from build123d import *

# Parameters (mm, degrees)
F2_SIZE        = 0.5
F4_DEPTH       = 2.5
F6_D           = 6.5
F6_CBORE_D     = 10.5
F6_CBORE_DEPTH = 5


with BuildPart() as f1:
    # F0 (on Top) → F1 (revolve)
    with BuildSketch(Plane.XY):
        with BuildLine():
            Line((-47.750211, -7.25), (-47.750212, -8))
            Line((-47.750212, -8), (-25.000581, -8))
            Line((-25.000581, -8), (-25, 0))
            Line((-25, 0), (-47.75, 0))
            Line((-47.75, 0), (-47.75019, -4))
            Line((-47.75019, -4), (-47.250211, -4))
            ThreePointArc((-47.250211, -4), (-46.189551, -4.43934), (-45.750211, -5.5))
            Line((-45.750211, -5.5), (-45.750211, -5.75))
            ThreePointArc((-45.750211, -5.75), (-46.189551, -6.81066), (-47.250211, -7.25))
            Line((-47.250211, -7.25), (-47.750211, -7.25))
        make_face()
    revolve(axis=Axis((0, 4.349666, 0), (0, 1, 0)))

    # F2
    f2_edges = [f1.edges().sort_by_distance(p)[0] for p in [
        (25.000581, -8, 0),
    ]]
    chamfer(f2_edges, length=F2_SIZE)

    # F3 (on face) → F4 (cut)
    with BuildSketch(Plane(origin=(0, 0, 0), x_dir=(-1, 0, 0), z_dir=(0, 1, 0))):
        with BuildLine():
            ThreePointArc((-4.265587, -23.938974), (-7.351028, -20.725712), (-10.56429, -23.811154))
            Line((-10.56429, -23.811154), (-11.035483, -47.030372))
            ThreePointArc((-11.035483, -47.030372), (-7.950042, -50.243634), (-4.73678, -47.158193))
            Line((-4.73678, -47.158193), (-4.265587, -23.938974))
        make_face()
    extrude(amount=-F4_DEPTH, mode=Mode.SUBTRACT)

    # F6 (through all)
    with Locations(Plane.XZ.offset(8)):
        with Locations((-28.85, 13.73333), (27.356101, 15.955209), (-0.6, -31.7)):
            CounterBoreHole(F6_D / 2, F6_CBORE_D / 2, F6_CBORE_DEPTH)


solid = f1.part
The listing builds one solid part. Answer for the finished solid, in the listing's coordinates (mm). A direction names the side the tool comes from. Coordinates: 2 decimals unless noted, no trailing zeros. Write each loop counter-clockwise with the first axis right and the second up, starting at its lowest first coordinate (ties: lowest second). Pieces come first, ordered by that corner, then holes. Notation, with made-up numbers: (49.25, 28) -> (87.25, 28) arc R8 cw to (87.25, 36) -> close; hole circle Ø9 at (83.25, 14.25). An arc over 180 degrees is marked (long way). One line per question, with ' | ' between items.
1. Which of the six approach directions +Z, -Z, +X, -X, +Y, -Y give full straight-line access (tool end or side, diameter ignored) to faces 1 (the flat face through (-21, -8, -21)), 2 (the cylindrical face through (32.206, -5.535, 13.944)), 3 (the flat face through (-46.2, -7.25, 10.8))?
Verdict:
face 1: +Z, -Z, +X, -X, -Y | face 2: -Y | face 3: none
2. For a pull along Y with two mould halves and no side action, classify faces 4 (the cylindrical face through (-23.842, -5.535, 15.31)), 5 (the flat face through (10.8, -4, 46.2)), 6 (the flat face through (21, 0, 22)) as released by +Y, released by -Y, zero draft, split by the parting line, or undercut.
Verdict:
face 4: zero draft | face 5: undercut | face 6: released by +Y
3. Section A-A (z = 0) is taken. Determine the outline of the cut face in (x, y).
Verdict:
outline: (-47.75, -8) -> (-25.5, -8) -> (-25, -7.5) -> (-25, 0) -> (-47.75, 0) -> (-47.75, -4) -> (-47.25, -4) arc R1.5 cw to (-45.75, -5.5) -> (-45.75, -5.75) arc R1.5 cw to (-47.25, -7.25) -> (-47.75, -7.25) -> close; (25, -7.5) -> (25.5, -8) -> (47.75, -8) -> (47.75, -7.25) -> (47.25, -7.25) arc R1.5 cw to (45.75, -5.75) -> (45.75, -5.5) arc R1.5 cw to (47.25, -4) -> (47.75, -4) -> (47.75, 0) -> (25, 0) -> close
4. Given pin 1 Ø1.5 at (y, z) = (-1.5, -15) entering from -X; pin 2 Ø3 at (x, y) = (24, -7) entering from +Z; pin 3 Ø3 at (x, z) = (0.5, -29.5) entering from -Y, each flat-ended and moving along its own axis, determine where each tip first touches the part or whether it passes through.
Verdict:
pin 1: stops at x = -45.57 | pin 2: stops at z = 42.11 | pin 3: stops at y = -3
5. Straight lines are drawn through the part: line 1 (Z direction, x = -0.6, y = -1.2); line 2 (Z direction, x = -0.6, y = -5.1); line 3 (Z direction, x = -15, y = -2.25). For each, find the intervals that lie inside material, in ascending order.
Verdict:
line 1: z = -47.75 to -34.95, -28.45 to -24.99, 24.99 to 47.75 | line 2: z = -45.8 to -36.95, -26.45 to -24.99, 24.99 to 45.8 | line 3: z = -45.33 to -20, 20 to 45.33
6. Section B-B (x = 0) is taken. State how many separate pieces and enclosed holes the cut face has, and give its area (3 significant figures).
Verdict:
separate pieces: 3 | enclosed holes: 0 | area: 281 mm^2
